Here's how the part is built. I have some questions about the finished solid (model axes, mm). A direction names the side the tool comes from. Round coordinates to 2 decimals unless told otherwise and drop trailing zeros. Order: outer loops, then holes, each group sorted by start corner. A loop starts at its lowest first (then second) coordinate and runs counter-clockwise, first axis right, second up. Notation, with made-up numbers: M 50,77 L 85,77 A19 cw 85,96 Z; hole C -25.5,-37 d1. An arc over 180 degrees is marked long. Answer as CSV lines item,"result". Start each with the question number.
```python
from build123d import *
from build123d.topology import SkipClean

# Parameters (mm, degrees)
F_2_BLOCK_BODY_DEPTH        = 7
AXLE_START                  = 24
SKETCH2_R                   = 3.7
AXLE_BODY_DEPTH             = 7.85
FAIRING_TOP_REACH           = 35.506
FAIRING_TOP_END_RADIUS      = 3.7
FAIRING_BOTTOM_DEPTH        = 38.2
FAIRING_SIDE_CUT_DEPTH      = 29.754999715
FAIRING_SIDE_CUT_DEPTH_BACK = 29.754999715
FAIRING_CORNER_REACH        = 43.353
FAIRING_CORNER_END_RADIUS   = 3.7
SKETCH6_W                   = 1.5
SKETCH6_H                   = 3.7
SKETCH3_W                   = 1.8
SKETCH3_H                   = 1.8
AXLE_CUT_DEPTH              = 7.85
FILLET1_R                   = 0.5
SKETCH7_R                   = 2.4
BLOCK_HOLES_DEPTH           = 7
SKETCH8_R                   = 3.1
SKETCH8_R_2                 = 2.4
RIM_CUTS_DEPTH              = 0.5
STOPPER_REACH               = 31.255
STOPPER_START_RADIUS        = 36.103557437
STOPPER_END_RADIUS          = 36.103557437
SKETCH9_W                   = 13
SKETCH9_H                   = 0.5
FILLET2_R                   = 1
FAIRING_MAIN_CUT_DEPTH      = 29.754999715
FAIRING_MAIN_CUT_DEPTH_BACK = 29.754999715
FILLET3_R                   = 5
FILLET4_R                   = 1


with BuildPart() as part:
    # Sketch1 → 2 Block Body (new body)
    with BuildSketch(Plane(origin=(0, 0, 0), x_dir=(1, 0, 0), z_dir=(0, 1, 0))):
        with BuildLine():
            Line((4, -3.7), (-4, -3.7))
            ThreePointArc((-4, -3.7), (-7.7, 0), (-4, 3.7))
            Line((-4, 3.7), (4, 3.7))
            ThreePointArc((4, 3.7), (7.7, 0), (4, -3.7))
        make_face()
    extrude(amount=-F_2_BLOCK_BODY_DEPTH)



with BuildPart() as body_2:
    # Sketch2 → Axle Body (new body)
    with BuildSketch(Plane(origin=(0, 0, 0), x_dir=(0, 0, -1), z_dir=(1, 0, 0)).offset(AXLE_START)):
        with BuildLine():
            ThreePointArc((3.7, -3.7), (0, -7.4), (-3.7, -3.7))
            Line((-3.7, -3.7), (-3.7, -10.2))
            Line((-3.7, -10.2), (3.7, -10.2))
            Line((3.7, -10.2), (3.7, -3.7))
        make_face()
        with Locations((0, -3.7)):
            Circle(SKETCH2_R)
    extrude(amount=-AXLE_BODY_DEPTH)


with BuildPart() as part_1:
    add(part.part)

    add(body_2.part)  # Fairing Top merges body 2
    # Fairing Top: up to this cylinder (the profile starts outside it)
    fairing_top_end = Plane(origin=(4, -1.781509, 0), z_dir=(0, 1, 0)) * Cylinder(FAIRING_TOP_END_RADIUS, 79.412, mode=Mode.PRIVATE)
    # Sketch4 → Fairing Top (add, up to the surface)
    with BuildSketch(Plane(origin=(24, 0, 0), x_dir=(0, 0, -1), z_dir=(1, 0, 0)), mode=Mode.PRIVATE) as fairing_top_sk1:
        with BuildLine():
            Line((0, -1.5), (0, 0))
            ThreePointArc((0, 0), (-2.61629509, -1.08370491), (-3.7, -3.7))
            Line((-3.7, -3.7), (-2.2, -3.7))
            ThreePointArc((-2.2, -3.7), (-1.555634919, -2.144365081), (0, -1.5))
        make_face()
    fairing_top_tool1 = extrude(fairing_top_sk1.sketch, amount=-FAIRING_TOP_REACH, mode=Mode.PRIVATE) - fairing_top_end
    add(fairing_top_tool1.solids().sort_by_distance((24, -1.781509, 1.918491))[0])

    # Sketch4<3> → Fairing Bottom (add)
    with BuildSketch(Plane(origin=(24, 0, 0), x_dir=(0, 0, -1), z_dir=(1, 0, 0))):
        with BuildLine():
            Line((-1.610057693, -10.2), (-3.133957759, -10.2))
            ThreePointArc((-3.133957759, -10.2), (-2.576502002, -12.823200932), (-1.833503605, -15.4))
            Line((-1.833503605, -15.4), (-0.407957853, -14.933288838))
            ThreePointArc((-0.407957853, -14.933288838), (-1.08913059, -12.586992982), (-1.610057693, -10.2))
        make_face()
        with BuildLine():
            Line((-2.2, -3.7), (-3.7, -3.7))
            ThreePointArc((-3.7, -3.7), (-3.558222165, -6.962299949), (-3.133957759, -10.2))
            Line((-3.133957759, -10.2), (-1.610057693, -10.2))
            ThreePointArc((-1.610057693, -10.2), (-2.052211942, -6.96335839), (-2.2, -3.7))
        make_face()
    extrude(amount=-FAIRING_BOTTOM_DEPTH)

    # Sketch5 → Fairing Side Cut (cut, two sides: drawn at the far end of the back side and taken through both)
    with SkipClean():  # the faces are left unmerged after this step: merging them gives an invalid solid
        with BuildSketch(Plane(origin=(0, 0, 0), x_dir=(0, 0, -1), z_dir=(1, 0, 0)).offset(-FAIRING_SIDE_CUT_DEPTH_BACK)):
            with BuildLine():
                Line((-1.833503605, -15.4), (-3.7, -15.4))
                Line((-3.7, -15.4), (-3.7, -3.7))
                ThreePointArc((-3.7, -3.7), (-3.230444229, -9.62397267), (-1.833503605, -15.4))
            make_face()
        extrude(amount=FAIRING_SIDE_CUT_DEPTH + FAIRING_SIDE_CUT_DEPTH_BACK, mode=Mode.SUBTRACT)

    # Fairing Corner: up to this cylinder (the profile starts outside it)
    fairing_corner_end = Plane(origin=(-4, -1.85, 0), z_dir=(0, 1, 0)) * Cylinder(FAIRING_CORNER_END_RADIUS, 95.106, mode=Mode.PRIVATE)
    # Sketch6 → Fairing Corner (add, up to the surface)
    with BuildSketch(Plane.ZY.offset(14.2), mode=Mode.PRIVATE) as fairing_corner_sk1:
        with Locations((2.95, -1.85)):
            Rectangle(SKETCH6_W, SKETCH6_H)
    fairing_corner_tool1 = extrude(fairing_corner_sk1.sketch, amount=-FAIRING_CORNER_REACH, mode=Mode.PRIVATE) - fairing_corner_end
    add(fairing_corner_tool1.solids().sort_by_distance((-14.2, -1.85, 2.95))[0])

    # Sketch3 → Axle Cut (cut)
    with BuildSketch(Plane(origin=(24, 0, 0), x_dir=(0, 0, -1), z_dir=(1, 0, 0))):
        with BuildLine():
            Line((-2.224859546, -4.6), (-0.9, -4.6))
            Line((-0.9, -4.6), (-0.9, -2.8))
            Line((-0.9, -2.8), (-2.224859546, -2.8))
            ThreePointArc((-2.224859546, -2.8), (-2.355808026, -3.24155857), (-2.4, -3.7))
            ThreePointArc((-2.4, -3.7), (-2.355808026, -4.15844143), (-2.224859546, -4.6))
        make_face()
        with BuildLine():
            Line((-0.9, -2.8), (0.9, -2.8))
            Line((0.9, -2.8), (0.9, -1.475140454))
            ThreePointArc((0.9, -1.475140454), (0.45844143, -1.344191974), (0, -1.3))
            ThreePointArc((0, -1.3), (-0.45844143, -1.344191974), (-0.9, -1.475140454))
            Line((-0.9, -1.475140454), (-0.9, -2.8))
        make_face()
        with Locations((0, -3.7)):
            Rectangle(SKETCH3_W, SKETCH3_H)
        with BuildLine():
            Line((0.9, -5.924859546), (0.9, -4.6))
            Line((0.9, -4.6), (-0.9, -4.6))
            Line((-0.9, -4.6), (-0.9, -5.924859546))
            ThreePointArc((-0.9, -5.924859546), (-0.45844143, -6.055808026), (0, -6.1))
            ThreePointArc((0, -6.1), (0.45844143, -6.055808026), (0.9, -5.924859546))
        make_face()
        with BuildLine():
            Line((0.9, -4.6), (2.224859546, -4.6))
            ThreePointArc((2.224859546, -4.6), (2.355808026, -4.15844143), (2.4, -3.7))
            ThreePointArc((2.4, -3.7), (2.355808026, -3.24155857), (2.224859546, -2.8))
            Line((2.224859546, -2.8), (0.9, -2.8))
            Line((0.9, -2.8), (0.9, -4.6))
        make_face()
        with BuildLine():
            Line((0.9, -7.288871689), (0.9, -6.1))
            Line((0.9, -6.1), (0, -6.1))
            Line((0, -6.1), (-0.9, -6.1))
            Line((-0.9, -6.1), (-0.9, -7.288871689))
            ThreePointArc((-0.9, -7.288871689), (0, -7.4), (0.9, -7.288871689))
        make_face()
        with BuildLine():
            Line((-0.9, -6.1), (0, -6.1))
            ThreePointArc((0, -6.1), (-0.45844143, -6.055808026), (-0.9, -5.924859546))
            Line((-0.9, -5.924859546), (-0.9, -6.1))
        make_face()
        with BuildLine():
            Line((0.9, -6.1), (0.9, -5.924859546))
            ThreePointArc((0.9, -5.924859546), (0.45844143, -6.055808026), (0, -6.1))
            Line((0, -6.1), (0.9, -6.1))
        make_face()
        with BuildLine():
            ThreePointArc((2.7, -6.229822128), (1.876271967, -6.888981578), (0.9, -7.288871689))
            ThreePointArc((0.9, -7.288871689), (0, -7.4), (-0.9, -7.288871689))
            ThreePointArc((-0.9, -7.288871689), (-1.876271967, -6.888981578), (-2.7, -6.229822128))
            Line((-2.7, -6.229822128), (-2.7, -9.170177872))
            ThreePointArc((-2.7, -9.170177872), (0, -8), (2.7, -9.170177872))
            Line((2.7, -9.170177872), (2.7, -6.229822128))
        make_face()
    extrude(amount=-AXLE_CUT_DEPTH, mode=Mode.SUBTRACT)

    # Fillet1
    # the kernel refuses this fillet: 0.5 mm, written as the material it adds along each edge
    with BuildSketch(Plane(origin=(24, -6.229822128, -2.7), x_dir=(0, -1, 0), z_dir=(-1, 0, 0))) as fillet1_piece_1:
        with BuildLine():
            CenterArc((1.047886636, 0.5), FILLET1_R, 148.411864495, 121.588135505)
            ThreePointArc((0.621968926, 0.761904762), (0.336413522, 0.36019377), (0, 0))
            Line((0, 0), (1.047886636, 0))
        make_face()
    extrude(amount=7.85)
    with BuildSketch(Plane(origin=(24, -9.170177872, -2.7), x_dir=(0, 0.6323800622573651, 0.7746582839287082), z_dir=(-1, 0, 0)), Plane(origin=(24, -6.229822128, 2.7), x_dir=(0, -0.6323800622573447, -0.7746582839287249), z_dir=(-1, 0, 0))) as fillet1_piece_2:
        with BuildLine():
            CenterArc((1.049991758, 0.495564032), FILLET1_R, 140.774061683, 121.588135505)
            Line((0.662662616, 0.811754063), (0, 0))
            ThreePointArc((0, 0), (0.491768292, 0.032826163), (0.983536583, 0))
        make_face()
    extrude(amount=7.85)
    with BuildSketch(Plane(origin=(24, -9.170177872, 2.7), x_dir=(0, 1, 0), z_dir=(-1, 0, 0))) as fillet1_piece_3:
        with BuildLine():
            CenterArc((1.047886636, 0.5), FILLET1_R, 148.411864495, 121.588135505)
            ThreePointArc((0.621968926, 0.761904762), (0.336413522, 0.36019377), (0, 0))
            Line((0, 0), (1.047886636, 0))
        make_face()
    extrude(amount=10.46971659)

    # Sketch7 → Block Holes (cut)
    with BuildSketch(Plane(origin=(0, 0, 0), x_dir=(1, 0, 0), z_dir=(0, 1, 0))):
        with Locations(Location((-4, 0, 0), (0, 0, 270))):
            Circle(SKETCH7_R)
        with Locations(Location((4, 0, 0), (0, 0, 270))):
            Circle(SKETCH7_R)
    extrude(amount=-BLOCK_HOLES_DEPTH, mode=Mode.SUBTRACT)

    # Sketch8 → Rim Cuts (cut)
    # profile 1 of 2: a face of its own
    with BuildSketch(Plane(origin=(0, 0, 0), x_dir=(1, 0, 0), z_dir=(0, 1, 0))):
        with Locations(Location((-4, 0, 0), (0, 0, 270))):
            Circle(SKETCH8_R)
        with Locations(Location((-4, 0, 0), (0, 0, 270))):
            Circle(SKETCH8_R_2, mode=Mode.SUBTRACT)
    # profile 2 of 2: a face of its own
    with BuildSketch(Plane(origin=(0, 0, 0), x_dir=(1, 0, 0), z_dir=(0, 1, 0))):
        with Locations(Location((4, 0, 0), (0, 0, 270))):
            Circle(SKETCH8_R)
        with Locations(Location((4, 0, 0), (0, 0, 270))):
            Circle(SKETCH8_R_2, mode=Mode.SUBTRACT)
    extrude(amount=-RIM_CUTS_DEPTH, mode=Mode.SUBTRACT)

    # Stopper: from a cylinder face, 31.255 long prism both ways, kept between that surface and its translate by the depth
    stopper_start = Plane(origin=(0, -3.7, -33.903557437), z_dir=(1, 0, 0)) * Cylinder(STOPPER_START_RADIUS, 135.717114875, mode=Mode.PRIVATE)
    stopper_end = Plane(origin=(0, -3.7, -34.403557437), z_dir=(1, 0, 0)) * Cylinder(STOPPER_END_RADIUS, 135.717114875, mode=Mode.PRIVATE)
    # Sketch9 → Stopper (add, from a surface)
    with BuildSketch(Plane.XY, mode=Mode.PRIVATE) as stopper_sk1:
        with Locations((0, -7.75)):
            Rectangle(SKETCH9_W, SKETCH9_H)
    stopper_tool1 = extrude(stopper_sk1.sketch, amount=STOPPER_REACH, both=True, mode=Mode.PRIVATE)
    add(((stopper_tool1 & stopper_start) - stopper_end).solids().sort_by_distance((0, -7.75, 1.72124))[0])

    # Fillet2
    fillet2_edges = [part_1.edges().sort_by_distance(p)[0] for p in [
        (24, -15.166644419, 1.120730729),
    ]]
    fillet(fillet2_edges, radius=FILLET2_R)

    # Sketch10 → Fairing Main Cut (cut, two sides: drawn at the far end of the back side and taken through both)
    with BuildSketch(Plane.XY.offset(-FAIRING_MAIN_CUT_DEPTH_BACK)):
        Polygon((-14.2, -3.8), (-14.2, 0), (-11.5, 0), align=None)
        Polygon((23, -15.4), (-10.2, -10.4), (-14.2, -3.8), (-14.2, -15.4), align=None)
    extrude(amount=FAIRING_MAIN_CUT_DEPTH + FAIRING_MAIN_CUT_DEPTH_BACK, mode=Mode.SUBTRACT)

    # Fillet3
    # the kernel refuses this fillet: 5 mm, written as the material it takes off along each edge
    with BuildSketch(Plane(origin=(24.982656407, -15.698592832, 2.745540381), x_dir=(-0.40943647865659716, 0.061662120279605645, 0.9102524665541475), z_dir=(-0.900102053497931, 0.1355575381773993, -0.41405367663153375))) as fillet3_piece_1:
        with BuildLine():
            CenterArc((FILLET3_R * 0.17621614345, FILLET3_R), FILLET3_R, 250.012318265, 19.987681735)
            Line((-FILLET3_R * 0.165601963428, FILLET3_R * 0.0602338685556), (-FILLET3_R * 0.172438325566, FILLET3_R * 0.0414385459267))
            Line((-FILLET3_R * 0.172438325566, FILLET3_R * 0.0414385459267), (-FILLET3_R * 0.003524322869, -FILLET3_R * 0.02))
            Line((-FILLET3_R * 0.003524322869, -FILLET3_R * 0.02), (FILLET3_R * 0.17621614345, -FILLET3_R * 0.02))
            Line((FILLET3_R * 0.17621614345, -FILLET3_R * 0.02), (FILLET3_R * 0.17621614345, 0))
        make_face()
    extrude(amount=7.848304428, mode=Mode.SUBTRACT)

    # Fillet4
    fillet4_edges = [part_1.edges().sort_by_distance(p)[0] for p in [
        (-11.5, 0, 2.95),
        (-10.2, -10.4, 2.335585217),
        (-14.2, -3.8, 2.949864271),
        (20.075, -10.2, -3.7),
    ]]
    fillet(fillet4_edges, radius=FILLET4_R)


solid = part_1.part
```
Item 1: If we section it at A-A on x = 12.5: Please give me the cut outline in (y, z).
Item 2: We'd pull the mould along Y, two halves only. Please class faces 5 (the flat face through (20, -4.6, -2)), 6 (the flat face through (-10, -2, 2.2)), 7 (the flat face through (2, -0.5, 2)): pulls with the +Y half, pulls with the -Y half, needs draft (parallel to the pull), parting line crosses it, or undercut.
Item 3: If we section it at B-B on y = -11.5: Please give me the cut outline in (x, z), and give its area (3 significant figures).
Item 4: Which directions (+Z, -Z, +X, -X, +Y, -Y) give clear straight access to the entire face, cutting with the end or side of a thin tool? Please do faces 1 (the flat face through (16.15, -2.4, 1.3)), 2 (the flat face through (12, -1, 0)), 3 (the cylindrical face through (6.024, -3.704, 1.29)), 4 (the flat face through (20, -4.6, 2)).
Item 5: If I drill on line 1 along X through (y, z) = (-4, 0); line 2 along Z through (x, y) = (-4, -3); line 3 along X through (y, z) = (-2, -2), over which ranges is the centre line in solid material (lowest first)?
Item 6: For P1, Ø2, axis at x = 3.5, z = -2, coming from the +Y side; P2, Ø1.2, axis at y = -2, z = 1, coming from the -X side; P3, Ø1, axis at x = -7, y = -10.5, coming from the +Z side, each with a flat end and sliding along its axis, tell me the tip position at first contact or that it passes through.
Geometry says:
1,outline,"M -13.82,0.75 A36.1 cw -3.7,2.2 A2.2 cw -1.5,0 L 0,0 A3.7 ccw -3.7,3.7 A37.6 ccw -13.82,2.31 Z"
2,face 5,"undercut"
2,face 6,"needs draft"
2,face 7,"pulls with the +Y half"
3,outline,"M -2.9,1.35 L 24,1.35 L 24,2.88 L -2.9,2.88 Z"
3,area,"41.3 mm²"
4,face 1,"-Z"
4,face 2,"-Z, +Y, -Y"
4,face 3,"+Y"
4,face 4,"+X"
5,line 1,"-7.7 to -6.4, -1.6 to 1.6, 6.4 to 7.7"
5,line 2,"-3.7 to -2.4, 2.4 to 3.7"
5,line 3,"-7.11 to -5.33, -2.67 to 2.67, 5.33 to 7.11, 16.15 to 24"
6,P1,"y = -0.5"
6,P2,"x = -7.68"
6,P3,"z = 3.17"
